The model under review builds one solid part; all positions refer to its coordinate system, in mm. A direction names the side the tool comes from. Give positions to 0.01 mm unless a question says otherwise; leave off trailing zeros. Order: outer loops, then holes, each group sorted by start corner. A loop starts at its lowest first (then second) coordinate and runs counter-clockwise, first axis right, second up. Notation, with made-up numbers: (-29, 11.5) - (18, 11.5) arc R13 cw to (18, 31.5) - close; hole circle Ø11 at (-29, -28). An arc over 180 degrees is marked (long way). Use CSV: the item, a comma, the result in double quotes. Start each with the question number.
1. Take a section at C-C, the plane y = -27.5. State the section outline as (x, z) points (3 decimals), then the cut area to 3 significant figures.
2. For pin 1 (2 mm diameter, centred on x = -19, z = 12.5, fed in from +Y); pin 2 (15 mm diameter, centred on x = 81, y = 11.5, fed in from -Z); pin 3 (14 mm diameter, centred on y = 9, z = 20.5, fed in from -X) (3 decimals); pin 4 (5 mm diameter, centred on x = 72.5, y = -28.5, fed in from -Z), all flat-tipped, find the tip position at first contact; note any pin that passes through.
3. Take a section at A-A, the plane y = -3. State the section outline as (x, z) points (3 decimals).
4. To check wall thickness, follow line 1 (X direction, y = -16, z = 2.5) (3 decimals); line 2 (Z direction, x = -14, y = -31.5) (3 decimals); line 3 (Y direction, x = 47, z = 40). State the ranges of each line that lie inside material, in increasing order. Write a range as [from, to].
5. Take a section at B-B, the plane z = -4. State the section outline as (x, y) points (3 decimals).
6. Machinability: for faces 1 (the flat face through (41.275, -1, 4)), 2 (the flat face through (60.325, 0, 41)), 3 (the flat face through (-5, -0.318, 31)), 4 (the cylindrical face through (31.85, 12.68, 51.21)), 5 (the flat face through (66, -25.4, 45)), which of the approach directions +Z, -Z, +X, -X, +Y, -Y give a long, thin tool a straight path to every point of the face, cutting with its end or side? Answer none if there is none.
7. Draft analysis for pull direction X (two halves, no side actions). For faces 6 (the cylindrical face through (31.85, -13.03, 51.21)), 7 (the cylindrical face through (57.475, -0.356, 62.055)), 8 (the flat face through (1, -32, 9.525)), state which applies: released by +X, released by -X, zero draft, split by the parting line, or undercut.
```python
from build123d import *

# Parameters (mm, degrees)
F1_DEPTH = 63.5
F2_DEPTH = 25.4
F3_DEPTH = 0.3175


with BuildPart() as f1:
    # F0 (on Front) → F1 (new body, symmetric)
    with BuildSketch(Plane.XZ):
        Polygon((41.275, -9.525), (41.275, 9.525), (22.225, 9.525), (-41.275, 9.525), (-41.275, -9.525), align=None)
    extrude(amount=F1_DEPTH, both=True)

    # F0 (on Front) → F2 (join, symmetric)
    with BuildSketch(Plane.XZ):
        with BuildLine():
            Line((22.225, 9.525), (41.275, 9.525))
            Line((41.275, 9.525), (41.275, 27.131808))
            ThreePointArc((41.275, 27.131808), (46.670684, 39.056554), (59.189906, 42.8752))
            Line((59.189906, 42.8752), (60.325, 42.8752))
            Line((60.325, 42.8752), (60.325, 61.9252))
            Line((60.325, 61.9252), (60.179103, 61.9252))
            ThreePointArc((60.179103, 61.9252), (57.43684, 62.05563), (54.692804, 61.970261))
            ThreePointArc((54.692804, 61.970261), (31.600311, 50.942919), (22.225, 27.131808))
            Line((22.225, 27.131808), (22.225, 9.525))
        make_face()
        Polygon((60.325, 61.9252), (60.325, 42.8752), (60.325, 38.1), (111.125, 38.1), (111.125, 66.675), (60.325, 66.675), align=None)
    extrude(amount=F2_DEPTH, both=True)

    # F0 (on Front) → F3 (join, symmetric)
    with BuildSketch(Plane.XZ):
        with BuildLine():
            Line((-41.275, 9.525), (22.225, 9.525))
            Line((22.225, 9.525), (22.225, 27.131808))
            ThreePointArc((22.225, 27.131808), (31.600311, 50.942919), (54.692804, 61.970261))
            add(Edge.make_bspline(
                [(-41.275, 9.525), (-38.055819, 41.44999), (20.570714, 64.283475), (54.692804, 61.970261)],
                knots=[0, 0, 0, 0, 109.36327, 109.36327, 109.36327, 109.36327], degree=3))
        make_face()
    extrude(amount=F3_DEPTH, both=True)


solid = f1.part
```
Determined:
1,outline,"(-41.275, -9.525) - (41.275, -9.525) - (41.275, 9.525) - (-41.275, 9.525) - close"
1,area,"1,570 mm²"
2,pin 1,"stops at y = 0.32"
2,pin 2,"stops at z = 38.1"
2,pin 3,"stops at x = 22.225"
2,pin 4,"passes through"
3,outline,"(-41.275, -9.525) - (41.275, -9.525) - (41.275, 27.132) arc R15.875 cw to (59.19, 42.875) - (60.325, 42.875) - (60.325, 38.1) - (111.125, 38.1) - (111.125, 66.675) - (60.325, 66.675) - (60.325, 61.925) - (60.179, 61.925) arc R34.925 ccw to (54.693, 61.97) arc R34.925 ccw to (22.225, 27.132) - (22.225, 9.525) - (-41.275, 9.525) - close"
4,line 1,"x = [-41.275, 41.275]"
4,line 2,"z = [-9.525, 9.525]"
4,line 3,"y = [-25.4, 25.4]"
5,outline,"(-41.275, -63.5) - (41.275, -63.5) - (41.275, 63.5) - (-41.275, 63.5) - close"
6,face 1,"-Z, +X, +Y, -Y"
6,face 2,"-Z, +Y, -Y"
6,face 3,"+Z, -X, -Y"
6,face 4,"+Z, -X, +Y"
6,face 5,"+Z, +X, -X, -Y"
7,face 6,"released by -X"
7,face 7,"undercut"
7,face 8,"zero draft"
